from build123d import *

# Parameters (mm, degrees)
F0_R     = 20
F2_DEPTH = 2.5
F3_DEPTH = 5
F4_DEPTH = 2.5
F5_R     = 1.5


with BuildPart() as f2:
    # F0 (on Top) → F2 (new body)
    with BuildSketch(Plane.XY):
        with Locations((30, 0)):
            Circle(F0_R)
        with BuildLine():
            ThreePointArc((20, 0), (24.4828773608, 0.5901820009), (28.6602540378, 2.3205080757))
            ThreePointArc((28.6602540378, 2.3205080757), (32.2474487139, 5.0730593618), (35, 8.6602540378))
            ThreePointArc((35, 8.6602540378), (35, -8.6602540378), (20, 0))
        make_face(mode=Mode.SUBTRACT)
        with BuildLine():
            ThreePointArc((24.9, 12.9903810568), (24.5784609691, 11.7903810568), (23.7, 10.9119200877))
            ThreePointArc((23.7, 10.9119200877), (20.4215390309, 14.1903810568), (24.9, 12.9903810568))
        make_face(mode=Mode.SUBTRACT)
    extrude(amount=F2_DEPTH)

    # F0 (on Top) → F3 (join)
    with BuildSketch(Plane.XY):
        with BuildLine():
            ThreePointArc((24.9, 12.9903810568), (20.4215390309, 14.1903810568), (23.7, 10.9119200877))
            ThreePointArc((23.7, 10.9119200877), (24.5784609691, 11.7903810568), (24.9, 12.9903810568))
        make_face()
        with BuildLine():
            ThreePointArc((35, 8.6602540378), (32.2474487139, 5.0730593618), (28.6602540378, 2.3205080757))
            ThreePointArc((28.6602540378, 2.3205080757), (24.4828773608, 0.5901820009), (20, 0))
            ThreePointArc((20, 0), (35, -8.6602540378), (35, 8.6602540378))
        make_face()
        with BuildLine():
            ThreePointArc((32, 0), (29, -1.7320508076), (29, 1.7320508076))
            ThreePointArc((29, 1.7320508076), (31, 1.7320508076), (32, 0))
        make_face(mode=Mode.SUBTRACT)
    extrude(amount=F3_DEPTH)

    # F1 (on Top) → F4 (join)
    with BuildSketch(Plane.XY):
        with BuildLine():
            Line((31.1749923535, 22.0351464548), (30, 20))
            ThreePointArc((30, 20), (32.6105238444, 19.8288972275), (35.1763809021, 19.3185165258))
            Line((35.1763809021, 19.3185165258), (34.5681601042, 21.5884274457))
            Line((34.5681601042, 21.5884274457), (32.8715762288, 21.8117869502))
            Line((32.8715762288, 21.8117869502), (31.1749923535, 22.0351464548))
        make_face()
        with BuildLine():
            Line((7.9648535452, 1.1749923535), (10, 0))
            Line((10, 0), (7.9648535452, -1.1749923535))
            Line((7.9648535452, -1.1749923535), (8.1882130498, -2.8715762288))
            Line((8.1882130498, -2.8715762288), (8.4115725543, -4.5681601042))
            Line((8.4115725543, -4.5681601042), (10.6814834742, -5.1763809021))
            Line((10.6814834742, -5.1763809021), (9.0197933522, -6.8380710241))
            Line((9.0197933522, -6.8380710241), (9.6746502848, -8.419035512))
            Line((9.6746502848, -8.419035512), (10.3295072173, -10))
            Line((10.3295072173, -10), (12.6794919243, -10))
            Line((12.6794919243, -10), (11.5044995708, -12.0351464548))
            Line((11.5044995708, -12.0351464548), (12.5462265136, -13.3927514382))
            Line((12.5462265136, -13.3927514382), (13.5879534564, -14.7503564216))
            Line((13.5879534564, -14.7503564216), (15.8578643763, -14.1421356237))
            Line((15.8578643763, -14.1421356237), (15.2496435784, -16.4120465436))
            Line((15.2496435784, -16.4120465436), (16.6072485618, -17.4537734864))
            Line((16.6072485618, -17.4537734864), (17.9648535452, -18.4955004292))
            Line((17.9648535452, -18.4955004292), (20, -17.3205080757))
            Line((20, -17.3205080757), (20, -19.6704927827))
            Line((20, -19.6704927827), (21.580964488, -20.3253497152))
            Line((21.580964488, -20.3253497152), (23.1619289759, -20.9802066478))
            Line((23.1619289759, -20.9802066478), (24.8236190979, -19.3185165258))
            Line((24.8236190979, -19.3185165258), (25.4318398958, -21.5884274457))
            Line((25.4318398958, -21.5884274457), (27.1284237712, -21.8117869502))
            Line((27.1284237712, -21.8117869502), (28.8250076465, -22.0351464548))
            Line((28.8250076465, -22.0351464548), (30, -20))
            Line((30, -20), (31.1749923535, -22.0351464548))
            Line((31.1749923535, -22.0351464548), (32.8715762288, -21.8117869502))
            Line((32.8715762288, -21.8117869502), (34.5681601042, -21.5884274457))
            Line((34.5681601042, -21.5884274457), (35.1763809021, -19.3185165258))
            Line((35.1763809021, -19.3185165258), (36.8380710241, -20.9802066478))
            Line((36.8380710241, -20.9802066478), (38.419035512, -20.3253497152))
            Line((38.419035512, -20.3253497152), (40, -19.6704927827))
            Line((40, -19.6704927827), (40, -17.3205080757))
            Line((40, -17.3205080757), (42.0351464548, -18.4955004292))
            Line((42.0351464548, -18.4955004292), (43.3927514382, -17.4537734864))
            Line((43.3927514382, -17.4537734864), (44.7503564216, -16.4120465436))
            Line((44.7503564216, -16.4120465436), (44.1421356237, -14.1421356237))
            Line((44.1421356237, -14.1421356237), (46.4120465436, -14.7503564216))
            Line((46.4120465436, -14.7503564216), (47.4537734864, -13.3927514382))
            Line((47.4537734864, -13.3927514382), (48.4955004292, -12.0351464548))
            Line((48.4955004292, -12.0351464548), (47.3205080757, -10))
            Line((47.3205080757, -10), (49.6704927827, -10))
            Line((49.6704927827, -10), (50.3253497152, -8.419035512))
            Line((50.3253497152, -8.419035512), (50.9802066478, -6.8380710241))
            Line((50.9802066478, -6.8380710241), (49.3185165258, -5.1763809021))
            Line((49.3185165258, -5.1763809021), (51.5884274457, -4.5681601042))
            Line((51.5884274457, -4.5681601042), (51.8117869502, -2.8715762288))
            Line((51.8117869502, -2.8715762288), (52.0351464548, -1.1749923535))
            Line((52.0351464548, -1.1749923535), (50, 0))
            Line((50, 0), (52.0351464548, 1.1749923535))
            Line((52.0351464548, 1.1749923535), (51.8117869502, 2.8715762288))
            Line((51.8117869502, 2.8715762288), (51.5884274457, 4.5681601042))
            Line((51.5884274457, 4.5681601042), (49.3185165258, 5.1763809021))
            Line((49.3185165258, 5.1763809021), (50.9802066478, 6.8380710241))
            Line((50.9802066478, 6.8380710241), (50.3253497152, 8.419035512))
            Line((50.3253497152, 8.419035512), (49.6704927827, 10))
            Line((49.6704927827, 10), (47.3205080757, 10))
            Line((47.3205080757, 10), (48.4955004292, 12.0351464548))
            Line((48.4955004292, 12.0351464548), (47.4537734864, 13.3927514382))
            Line((47.4537734864, 13.3927514382), (46.4120465436, 14.7503564216))
            Line((46.4120465436, 14.7503564216), (44.1421356237, 14.1421356237))
            Line((44.1421356237, 14.1421356237), (44.7503564216, 16.4120465436))
            Line((44.7503564216, 16.4120465436), (43.3927514382, 17.4537734864))
            Line((43.3927514382, 17.4537734864), (42.0351464548, 18.4955004292))
            Line((42.0351464548, 18.4955004292), (40, 17.3205080757))
            Line((40, 17.3205080757), (40, 19.6704927827))
            Line((40, 19.6704927827), (38.419035512, 20.3253497152))
            Line((38.419035512, 20.3253497152), (36.8380710241, 20.9802066478))
            Line((36.8380710241, 20.9802066478), (35.1763809021, 19.3185165258))
            ThreePointArc((35.1763809021, 19.3185165258), (32.6105238444, 19.8288972275), (30, 20))
            Line((30, 20), (28.8250076465, 22.0351464548))
            Line((28.8250076465, 22.0351464548), (27.1284237712, 21.8117869502))
            Line((27.1284237712, 21.8117869502), (25.4318398958, 21.5884274457))
            Line((25.4318398958, 21.5884274457), (24.8236190979, 19.3185165258))
            Line((24.8236190979, 19.3185165258), (23.1619289759, 20.9802066478))
            Line((23.1619289759, 20.9802066478), (21.580964488, 20.3253497152))
            Line((21.580964488, 20.3253497152), (20, 19.6704927827))
            Line((20, 19.6704927827), (20, 17.3205080757))
            Line((20, 17.3205080757), (17.9648535452, 18.4955004292))
            Line((17.9648535452, 18.4955004292), (16.6072485618, 17.4537734864))
            Line((16.6072485618, 17.4537734864), (15.2496435784, 16.4120465436))
            Line((15.2496435784, 16.4120465436), (15.8578643763, 14.1421356237))
            Line((15.8578643763, 14.1421356237), (13.5879534564, 14.7503564216))
            Line((13.5879534564, 14.7503564216), (12.5462265136, 13.3927514382))
            Line((12.5462265136, 13.3927514382), (11.5044995708, 12.0351464548))
            Line((11.5044995708, 12.0351464548), (12.6794919243, 10))
            Line((12.6794919243, 10), (10.3295072173, 10))
            Line((10.3295072173, 10), (9.6746502848, 8.419035512))
            Line((9.6746502848, 8.419035512), (9.0197933522, 6.8380710241))
            Line((9.0197933522, 6.8380710241), (10.6814834742, 5.1763809021))
            Line((10.6814834742, 5.1763809021), (8.4115725543, 4.5681601042))
            Line((8.4115725543, 4.5681601042), (8.1882130498, 2.8715762288))
            Line((8.1882130498, 2.8715762288), (7.9648535452, 1.1749923535))
        make_face()
        with BuildLine():
            ThreePointArc((32, 0), (30, -2), (28, 0))
            ThreePointArc((28, 0), (30, 2), (32, 0))
        make_face(mode=Mode.SUBTRACT)
    extrude(amount=F4_DEPTH)

    # F5
    f5_edges = [f2.edges().sort_by_distance(p)[0] for p in [
        (20, 0, 3.75),
        (35, 8.660254, 3.75),
    ]]
    fillet(f5_edges, radius=F5_R)


solid = f2.part
Verification items for the finished model (mm, model axes). A direction names the side the tool comes from. Coordinates: 2 decimals unless noted, no trailing zeros. Order: outer loops, then holes, each group sorted by start corner. A loop starts at its lowest first (then second) coordinate and runs counter-clockwise, first axis right, second up. Notation, with made-up numbers: M 16,-16.5 L 71,-16.5 A22 ccw 71,-8.5 Z; hole C 13.5,-6 d6. An arc over 180 degrees is marked long. One line per item, written item: value. Start each with the question number.
Item 1: Sectioned sample at B-B on y = 13.5. Record the cut outline in (x, z), then the cut area to 3 significant figures.
Item 2: Sectioned sample at A-A on x = 39. Record the cut outline in (y, z), then the cut area to 3 significant figures.
Item 3: Depth check by flat-ended pin: P1, Ø4, axis at x = 26.5, y = 4.5, coming from the +Z side; P2, Ø2.5, axis at x = 48.5, z = 1.5, coming from the -Y side; P3, Ø0.7, axis at y = 18.5, z = 1.5, coming from the +X side. Enter the tip coordinate at first touch or a pass-through.
Item 4: Mould release check, pull along X, two halves, no side actions. Record for faces 5 (the flat face through (19, -17.9, 1.2)), 6 (the flat face through (43.41, 17.44, 1.23)), 7 (the flat face through (16.59, -17.44, 1.23)), 8 (the flat face through (36.02, 20.16, 1.23)): pulls with the +X half, pulls with the -X half, needs draft (parallel to the pull), parting line crosses it, or undercut.
Item 5: Thickness scan on probe 1 along Y at (x, z) = (11, 1.5); probe 2 along Y at (x, z) = (30, 3); probe 3 along Z at (x, y) = (13.5, 8). Record the ranges inside material, lowest first.
Item 6: Sectioned sample at C-C on x = 22.5. Record the cut outline in (y, z).
Item 7: Sectioned sample at D-D on x = 16.5. Record the cut outline in (y, z), then the cut area to 3 significant figures.
Item 8: Access from +Z, -Z, +X, -X, +Y, -Y to the whole of each face (thin tool, end or side, straight path). Record for faces 1 (the flat face through (45.26, -14.44, 1.23)), 2 (the flat face through (16.63, 17.47, 1.23)), 3 (the flat face through (9.562, 4.877, 1.232)), 4 (the flat face through (19, 17.9, 1.2)).
Calculated:
1. outline: M 12.63,0 L 47.37,0 L 47.37,2.5 L 24.85,2.5 L 24.85,5 L 20.15,5 L 20.15,2.5 L 12.63,2.5 Z
1. area: 98.6 mm^2
2. outline: M -20.08,0 L 20.08,0 L 20.08,2.5 L 4.36,2.5 L 4.36,5 L -4.36,5 L -4.36,2.5 L -20.08,2.5 Z
2. area: 122 mm^2
3. P1: z = 2.5
3. P2: y = -13.66
3. P3: x = 42.49
4. face 5: undercut
4. face 6: pulls with the +X half
4. face 7: pulls with the -X half
4. face 8: undercut
5. probe 1: -10 to 10
5. probe 2: -10 to -2, 2 to 3.18
5. probe 3: 0 to 2.5
6. outline: M -20.71,0 L 20.71,0 L 20.71,2.5 L 15.39,2.5 L 15.39,5 L 10.59,5 L 10.59,2.5 L 0.18,2.5 L 0.18,5 L -6.61,5 L -6.61,2.5 L -20.71,2.5 Z
7. outline: M -17.37,0 L 17.37,0 L 17.37,2.5 L -17.37,2.5 Z
7. area: 86.9 mm^2
8. face 1: +Z, -Z
8. face 2: +Z, -Z, -X, +Y
8. face 3: +Z, -Z, -X
8. face 4: +Z, -Z, +Y
